from build123d import *

# Parameters (mm, degrees)
SKETCH1_W                                 = 16
SKETCH1_H                                 = 16
BASE_DEPTH                                = 50
SKETCH2_W                                 = 2
SKETCH2_H                                 = 16
RODSLOT_DEPTH                             = 54.103672189
F_5_1_5_1_FREE_HOLE_FOR_SCREW_D           = 5.1
F_5_1_5_1_FREE_HOLE_FOR_SCREW_DEPTH       = 7.5
F_5_1_5_1_FREE_HOLE_FOR_SCREW_CSINK_D     = 6.1
F_5_1_5_1_FREE_HOLE_FOR_SCREW_CSINK_ANGLE = 90
F_5_1_5_1_FREE_HOLE_FOR_SCREW_TIP         = 1.056244584
M5X0_8_TAPPED_HOLE_FOR_ROD_SCREW_D        = 4.2
M5X0_8_TAPPED_HOLE_FOR_ROD_SCREW_DEPTH    = 7.6381927
M5X0_8_TAPPED_HOLE_FOR_ROD_SCREW_TIP      = 1.2618073
F_3_1_3_1_SCREW_HOLES_D                   = 2.5
F_10_2_10_2_ROD_HOLE_D                    = 10.2


with BuildPart() as part:
    # Sketch1 → Base (new body)
    with BuildSketch(Plane.XY):
        Rectangle(SKETCH1_W, SKETCH1_H)
    extrude(amount=BASE_DEPTH)

    # Sketch2 → RodSlot (cut, through all)
    with BuildSketch(Plane(origin=(0, 8, 0), x_dir=(1, 0, 0), z_dir=(0, 1, 0))):
        with Locations((0, -42)):
            Rectangle(SKETCH2_W, SKETCH2_H)
    extrude(amount=-RODSLOT_DEPTH, mode=Mode.SUBTRACT)

    # Ø5.1 (5.1) free hole for screw
    with Locations(Plane(origin=(8, 0, 0), x_dir=(0, 0, -1), z_dir=(1, 0, 0))):
        with Locations((-45, 0)):
            CounterSinkHole(F_5_1_5_1_FREE_HOLE_FOR_SCREW_D / 2, F_5_1_5_1_FREE_HOLE_FOR_SCREW_CSINK_D / 2, depth=F_5_1_5_1_FREE_HOLE_FOR_SCREW_DEPTH, counter_sink_angle=F_5_1_5_1_FREE_HOLE_FOR_SCREW_CSINK_ANGLE)
            with Locations((0, 0, -(F_5_1_5_1_FREE_HOLE_FOR_SCREW_DEPTH + F_5_1_5_1_FREE_HOLE_FOR_SCREW_TIP / 2))):  # 135° drill point
                Cone(0, F_5_1_5_1_FREE_HOLE_FOR_SCREW_D / 2, F_5_1_5_1_FREE_HOLE_FOR_SCREW_TIP, mode=Mode.SUBTRACT)

    # M5x0.8 Tapped Hole for rod screw
    with Locations(Plane.ZY.offset(8)):
        with Locations((45, 0)):
            Hole(M5X0_8_TAPPED_HOLE_FOR_ROD_SCREW_D / 2, depth=M5X0_8_TAPPED_HOLE_FOR_ROD_SCREW_DEPTH)
            with Locations((0, 0, -(M5X0_8_TAPPED_HOLE_FOR_ROD_SCREW_DEPTH + M5X0_8_TAPPED_HOLE_FOR_ROD_SCREW_TIP / 2))):  # 118° drill point
                Cone(0, M5X0_8_TAPPED_HOLE_FOR_ROD_SCREW_D / 2, M5X0_8_TAPPED_HOLE_FOR_ROD_SCREW_TIP, mode=Mode.SUBTRACT)

    # Ø3.1 (3.1) screw holes (through all)
    with Locations(Plane.YZ.offset(8)):
        with Locations((3, 5), (-3, 11)):
            Hole(F_3_1_3_1_SCREW_HOLES_D / 2)

    # Ø10.2 (10.2) Rod Hole (through all)
    with Locations(Plane(origin=(0, 8, 0), x_dir=(1, 0, 0), z_dir=(0, 1, 0))):
        with Locations((0, -30)):
            Hole(F_10_2_10_2_ROD_HOLE_D / 2)


solid = part.part
Source: CAD feature listing. Evaluate the final solid. Frame: model axes, mm. A direction names the side the tool comes from. Give positions to 0.01 mm unless a question says otherwise; leave off trailing zeros. Write each loop counter-clockwise with the first axis right and the second up, starting at its lowest first coordinate (ties: lowest second). Pieces come first, ordered by that corner, then holes. Notation, with made-up numbers: M -25.5,-3.75 L -2.5,-3.75 A3 ccw -2.5,1.25 Z; hole C 83,64.25 d11. An arc over 180 degrees is marked long. Answer as a JSON object with one key per item and string values.
Q1. Access query for faces 1 (the face through (4.204, 0.112, 42.452)), 2 (the face through (1, 0, 41)), 3 (the face through (-0.112, 2.423, 3.891)). Directions: +Z, -Z, +X, -X, +Y, -Y. A direction counts if a zero-diameter tool reaches every point of the face in a straight line with its end or side. Return the directions, or none.
Geometry check:
{"face 1": "+X", "face 2": "+Z, +Y, -Y", "face 3": "+X, -X"}
Q2. Mould query, pull axis X, two halves, no side actions, for faces 4 (the face through (-5, 0, 50)), 5 (the face through (-1, 0.1, 42.6)), 6 (the face through (8, 0, 25)). Classes: +X half, -X half, draft (parallel to the pull), parting line (faces both ways), or undercut.
Geometry check:
{"face 4": "draft", "face 5": "undercut", "face 6": "+X half"}
Q3. Cut plane A-A, the plane x = -4.5. Return the cut outline in (y, z), then the cut area to 3 significant figures.
Geometry check:
{"outline": "M -8,0 L 8,0 L 8,27.6 L -8,27.6 Z; M -8,32.4 L 8,32.4 L 8,50 L -8,50 Z; hole C -3,11 d2.5; hole C 0,45 d4.2; hole C 3,5 d2.5", "area": "700 mm^2"}
Q4. Cut plane C-C, the plane z = 30. Return the cut outline in (x, y), then the cut area to 3 significant figures.
Geometry check:
{"outline": "M -8,-8 L -5.1,-8 L -5.1,8 L -8,8 Z; M 5.1,-8 L 8,-8 L 8,8 L 5.1,8 Z", "area": "92.8 mm^2"}
Q5. Cut plane D-D, the plane x = 6.75. Return the cut outline in (y, z), then the cut area to 3 significant figures.
Geometry check:
{"outline": "M -8,0 L 8,0 L 8,50 L -8,50 Z; hole C -3,11 d2.5; hole C 0,45 d5.1; hole C 3,5 d2.5", "area": "770 mm^2"}
Q6. Ray query, line 1 along X through (y, z) = (5.75, 36); line 2 along Z through (x, y) = (-2.75, 2.25); line 3 along X through (y, z) = (4.5, 30). Return the intervals inside material, ascending.
Geometry check:
{"line 1": "x = -8 to -1, 1 to 8", "line 2": "z = 0 to 4, 6 to 25.7, 34.3 to 50", "line 3": "x = -8 to -5.1, 5.1 to 8"}
Q7. Cut plane B-B, the plane y = 0. Return the cut outline in (x, z).
Geometry check:
{"outline": "M -8,0 L 8,0 L 8,41.95 L 7.5,42.45 L 1,42.45 L 1,35 A5.1 cw long -1,35 L -1,42.9 L -8,42.9 Z; M -8,47.1 L -1,47.1 L -1,50 L -8,50 Z; M 1,47.55 L 7.5,47.55 L 8,48.05 L 8,50 L 1,50 Z"}
Q8. Contact query for a flat-ended pin moving along its axis: P1, Ø3, axis at y = 3, z = 5, coming from the -X side. Output: stop coordinate, or through.
Geometry check:
{"P1": "stops at x = -8"}
